Design review of the part built by this model. Coordinates are the model's own, in mm. A direction names the side the tool comes from. Round coordinates to 2 decimals unless told otherwise and drop trailing zeros. Write each loop counter-clockwise with the first axis right and the second up, starting at its lowest first coordinate (ties: lowest second). Pieces come first, ordered by that corner, then holes. Notation, with made-up numbers: M 58,41 L 72,41 A31 cw 72,72 Z; hole C 4,-14 d5. An arc over 180 degrees is marked long. Use CSV: the item, a comma, the result in double quotes.
from build123d import *

# Parameters (mm, degrees)
SKETCH1_W                    = 8.5
SKETCH1_H                    = 4
SKETCH2_W                    = 5
SKETCH2_H                    = 5
BOSS_EXTRUDE1_DEPTH          = 4.5
SKETCH3_R                    = 3
BOSS_EXTRUDE2_DEPTH          = 6
SKETCH8_W                    = 2.5
SKETCH8_H                    = 6.839743052
CUT_EXTRUDE2_DEPTH           = 2
FILLET1_R                    = 1
M3X0_5_TAPPED_HOLE1_D        = 2.5
M3X0_5_TAPPED_HOLE1_DEPTH    = 7.5
M3X0_5_TAPPED_HOLE1_TIP      = 0.751075774
M2_5X0_45_TAPPED_HOLE2_D     = 2.05
M2_5X0_45_TAPPED_HOLE2_DEPTH = 5
M2_5X0_45_TAPPED_HOLE2_TIP   = 0.615882135


with BuildPart() as part:
    # Sketch1 → Revolve1 (revolve)
    with BuildSketch(Plane.XY, mode=Mode.PRIVATE) as revolve1_sk:
        with Locations((9.25, 2)):
            Rectangle(SKETCH1_W, SKETCH1_H)
    revolve(revolve1_sk.sketch.rotate(Axis((5, 0, 0), (1, 0, 0)), 270), axis=Axis((5, 0, 0), (1, 0, 0)))

    # Sketch2 → Boss-Extrude1 (add)
    with BuildSketch(Plane.ZY.offset(-5)):
        Rectangle(SKETCH2_W, SKETCH2_H)
    extrude(amount=BOSS_EXTRUDE1_DEPTH)

    # Sketch3 → Boss-Extrude2 (add)
    with BuildSketch(Plane(origin=(13.5, 0, 0), x_dir=(0, 0, -1), z_dir=(1, 0, 0))):
        Circle(SKETCH3_R)
    extrude(amount=BOSS_EXTRUDE2_DEPTH)

    # Sketch8 → Cut-Extrude2 (cut)
    with BuildSketch(Plane(origin=(19.5, 0, 0), x_dir=(0, 0, -1), z_dir=(1, 0, 0))):
        Rectangle(SKETCH8_W, SKETCH8_H)
    extrude(amount=-CUT_EXTRUDE2_DEPTH, mode=Mode.SUBTRACT)

    # Fillet1
    fillet1_edges = [part.edges().sort_by_distance(p)[0] for p in [
        (2.75, -2.5, 2.5),
        (2.75, 2.5, 2.5),
        (2.75, 2.5, -2.5),
        (2.75, -2.5, -2.5),
    ]]
    fillet(fillet1_edges, radius=FILLET1_R)

    # M3x0.5 Tapped Hole1
    with Locations(Plane(origin=(0.5, 0, 0), x_dir=(0, 0, -1), z_dir=(-1, 0, 0))):
        with Locations((0, 0)):
            Hole(M3X0_5_TAPPED_HOLE1_D / 2, depth=M3X0_5_TAPPED_HOLE1_DEPTH)
            with Locations((0, 0, -(M3X0_5_TAPPED_HOLE1_DEPTH + M3X0_5_TAPPED_HOLE1_TIP / 2))):  # 118° drill point
                Cone(0, M3X0_5_TAPPED_HOLE1_D / 2, M3X0_5_TAPPED_HOLE1_TIP, mode=Mode.SUBTRACT)

    # M2.5x0.45 Tapped Hole2
    with Locations(Plane(origin=(17.5, 0, 0), x_dir=(0, 0, 1), z_dir=(1, 0, 0))):
        with Locations((0, 0)):
            Hole(M2_5X0_45_TAPPED_HOLE2_D / 2, depth=M2_5X0_45_TAPPED_HOLE2_DEPTH)
            with Locations((0, 0, -(M2_5X0_45_TAPPED_HOLE2_DEPTH + M2_5X0_45_TAPPED_HOLE2_TIP / 2))):  # 118° drill point
                Cone(0, M2_5X0_45_TAPPED_HOLE2_D / 2, M2_5X0_45_TAPPED_HOLE2_TIP, mode=Mode.SUBTRACT)


solid = part.part
1) Add section A-A on x = 2.5. Write out the cut boundary in (y, z), then the cut area to 3 significant figures.
Answers:
outline,"M -2.5,-1.5 A1 ccw -1.5,-2.5 L 1.5,-2.5 A1 ccw 2.5,-1.5 L 2.5,1.5 A1 ccw 1.5,2.5 L -1.5,2.5 A1 ccw -2.5,1.5 Z; hole C 0,0 d2.5"
area,"19.2 mm²"
2) Add section C-C on z = -2.75. Write out the cut boundary in (x, y), then the cut area to 3 significant figures.
Answers:
outline,"M 5,-2.9 L 13.5,-2.9 L 13.5,-1.2 L 19.5,-1.2 L 19.5,1.2 L 13.5,1.2 L 13.5,2.9 L 5,2.9 Z"
area,"63.8 mm²"
3) Wall thickness on line 1 along Y through (x, z) = (3.5, 0); line 2 along X through (y, z) = (-1.5, -1); line 3 along X through (y, z) = (1.75, 2.5): over which ranges is each line inside the solid? List them lowest first. Write a range as [from, to].
Answers:
line 1,"[-2.5, -1.25], [1.25, 2.5]"
line 2,"[0.5, 17.5]"
line 3,"[5, 13.5]"
4) The part is to be moulded in two halves that separate along Y. For faces 5 (the face through (3, 2.5, 0)), 6 (the face through (8.62, 0.21, 0.05)), 7 (the face through (13.5, 3, 1)), 8 (the face through (3, -2.5, 0)), say which applies: released by +Y, released by -Y, zero draft, split by the parting line, or undercut.
Answers:
face 5,"released by +Y"
face 6,"undercut"
face 7,"zero draft"
face 8,"released by -Y"
5) For pin 1 Ø1.5 at (x, y) = (4, 0.5) entering from +Z; pin 2 Ø4 at (y, z) = (0, 0.5) entering from +X; pin 3 Ø2 at (y, z) = (0, 0) entering from -X; pin 4 Ø1.5 at (x, y) = (3.5, -0.5) entering from -Z, all flat-tipped, find the tip position at first contact; note any pin that passes through.
Answers:
pin 1,"z = 2.5"
pin 2,"x = 19.5"
pin 3,"x = 8.15"
pin 4,"z = -2.5"
6) Add section B-B on z = 1.75. Write out the cut boundary in (x, y).
Answers:
outline,"M 0.5,-2.47 L 5,-2.47 L 5,-3.6 L 13.5,-3.6 L 13.5,-2.44 L 19.5,-2.44 L 19.5,2.44 L 13.5,2.44 L 13.5,3.6 L 5,3.6 L 5,2.47 L 0.5,2.47 Z"
7) Add section D-D on x = 8.25. Write out the cut boundary in (y, z).
Answers:
outline,"C 0,0 d8; hole C 0,0 d1.67"
8) Machinability: for faces 1 (the face through (16.46, -1.15, -2.77)), 2 (the face through (5, 0, 3)), 3 (the face through (3, 0, 2.5)), 4 (the face through (17.5, 1, -1)), which of the approach directions +Z, -Z, +X, -X, +Y, -Y give a long, thin tool a straight path to every point of the face, cutting with its end or side? Answer none if there is none.
Answers:
face 1,"+X"
face 2,"-X"
face 3,"+Z, -X, +Y, -Y"
face 4,"+X, +Y, -Y"
